Input: dimensioned drawing with shaded views. Units: mm. Origin: part minimum x, y, z. A direction names the side the tool comes from. Give positions to 0.01 mm unless a question says otherwise; leave off trailing zeros. Write each loop counter-clockwise with the first axis right and the second up, starting at its lowest first coordinate (ties: lowest second). Pieces come first, ordered by that corner, then holes.
Q1. Section C-C (z = 45). Return the cut outline in (x, y), plus the area to 3 significant figures.
Q2. Reachability of the marked faces 1 and 2 from +Z, -Z, +X, -X, +Y, -Y: full face, straight path, thin tool, end or side. Return the list, or none.
Q3. Section D-D (y = 58). Return the cut outline in (x, z).
Q4. Line query: line 1 (Z direction, x = 64.5, y = 21); line 2 (Y direction, x = 40.5, z = 23). Output: solid intervals per line, ascending.
Q5. Section A-A (x = 38.1). Return the cut outline in (y, z), plus the area to 3 significant figures.
Q6. Pin query (flat end, axial travel): pin 1 Ø3 at (x, y) = (10, 65) entering from +Z; pin 2 Ø10 at (x, z) = (33.5, 80) entering from +Y; pin 3 Ø6 at (y, z) = (30, 16) entering from +X. Return the tip coordinate at first contact, or that it passes through.
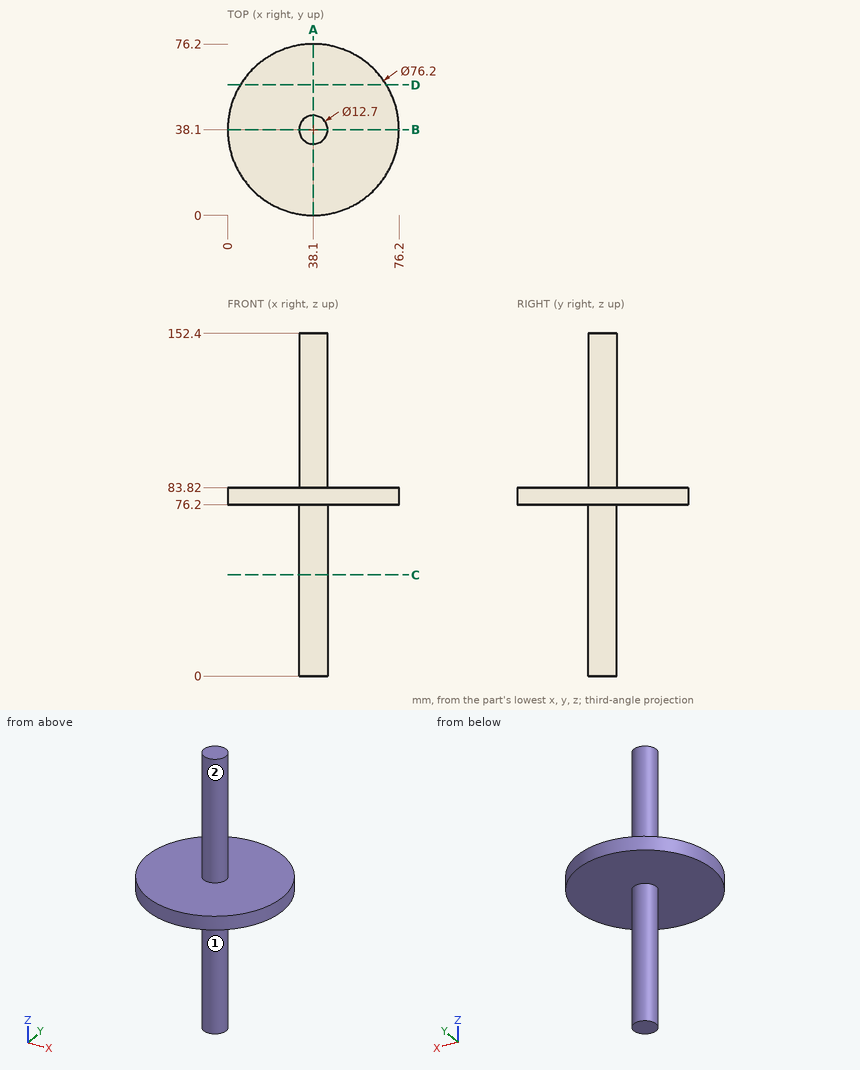
Computed:
1. outline: circle Ø12.7 at (38.1, 38.1)
1. area: 127 mm2
2. face 1: -Z
2. face 2: +Z
3. outline: (5.61, 76.2) - (70.59, 76.2) - (70.59, 83.82) - (5.61, 83.82) - close
4. line 1: z = 76.2 to 83.82
4. line 2: y = 32.22 to 43.98
5. outline: (0, 76.2) - (31.75, 76.2) - (31.75, 0) - (44.45, 0) - (44.45, 76.2) - (76.2, 76.2) - (76.2, 83.82) - (44.45, 83.82) - (44.45, 152.4) - (31.75, 152.4) - (31.75, 83.82) - (0, 83.82) - close
5. area: 2,420 mm2
6. pin 1: stops at z = 83.82
6. pin 2: stops at y = 76.2
6. pin 3: stops at x = 41.88
